```python
from build123d import *

# Parameters (mm, degrees)
SKETCH_1_W          = 300
SKETCH_1_H          = 200
EXTRUDE_1_DEPTH     = 5
SKETCH_3_R          = 1.5
SKETCH_3_R_2        = 2.5
CUT_EXTRUDE_1_DEPTH = 181.346887969


with BuildPart() as part:
    # 草圖1 → 填料-伸長1 (new body)
    with BuildSketch(Plane(origin=(0, 0, 0), x_dir=(1, 0, 0), z_dir=(0, 1, 0))):
        Rectangle(SKETCH_1_W, SKETCH_1_H)
        with BuildLine():
            Line((-137.5, 92.5), (-137.5, 87.5))
            ThreePointArc((-137.5, 87.5), (-140, 85), (-142.5, 87.5))
            Line((-142.5, 87.5), (-142.5, 92.5))
            ThreePointArc((-142.5, 92.5), (-140, 95), (-137.5, 92.5))
        make_face(mode=Mode.SUBTRACT)
        with BuildLine():
            Line((-137.5, 66.785714286), (-137.5, 61.785714286))
            ThreePointArc((-137.5, 61.785714286), (-140, 59.285714286), (-142.5, 61.785714286))
            Line((-142.5, 61.785714286), (-142.5, 66.785714286))
            ThreePointArc((-142.5, 66.785714286), (-140, 69.285714286), (-137.5, 66.785714286))
        make_face(mode=Mode.SUBTRACT)
        with BuildLine():
            Line((-137.5, 41.071428571), (-137.5, 36.071428571))
            ThreePointArc((-137.5, 36.071428571), (-140, 33.571428571), (-142.5, 36.071428571))
            Line((-142.5, 36.071428571), (-142.5, 41.071428571))
            ThreePointArc((-142.5, 41.071428571), (-140, 43.571428571), (-137.5, 41.071428571))
        make_face(mode=Mode.SUBTRACT)
        with BuildLine():
            Line((-137.5, 15.357142857), (-137.5, 10.357142857))
            ThreePointArc((-137.5, 10.357142857), (-140, 7.857142857), (-142.5, 10.357142857))
            Line((-142.5, 10.357142857), (-142.5, 15.357142857))
            ThreePointArc((-142.5, 15.357142857), (-140, 17.857142857), (-137.5, 15.357142857))
        make_face(mode=Mode.SUBTRACT)
        with BuildLine():
            Line((-137.5, -10.357142857), (-137.5, -15.357142857))
            ThreePointArc((-137.5, -15.357142857), (-140, -17.857142857), (-142.5, -15.357142857))
            Line((-142.5, -15.357142857), (-142.5, -10.357142857))
            ThreePointArc((-142.5, -10.357142857), (-140, -7.857142857), (-137.5, -10.357142857))
        make_face(mode=Mode.SUBTRACT)
        with BuildLine():
            Line((-137.5, -36.071428571), (-137.5, -41.071428571))
            ThreePointArc((-137.5, -41.071428571), (-140, -43.571428571), (-142.5, -41.071428571))
            Line((-142.5, -41.071428571), (-142.5, -36.071428571))
            ThreePointArc((-142.5, -36.071428571), (-140, -33.571428571), (-137.5, -36.071428571))
        make_face(mode=Mode.SUBTRACT)
        with BuildLine():
            Line((-137.5, -61.785714286), (-137.5, -66.785714286))
            ThreePointArc((-137.5, -66.785714286), (-140, -69.285714286), (-142.5, -66.785714286))
            Line((-142.5, -66.785714286), (-142.5, -61.785714286))
            ThreePointArc((-142.5, -61.785714286), (-140, -59.285714286), (-137.5, -61.785714286))
        make_face(mode=Mode.SUBTRACT)
        with BuildLine():
            Line((-137.5, -87.5), (-137.5, -92.5))
            ThreePointArc((-137.5, -92.5), (-140, -95), (-142.5, -92.5))
            Line((-142.5, -92.5), (-142.5, -87.5))
            ThreePointArc((-142.5, -87.5), (-140, -85), (-137.5, -87.5))
        make_face(mode=Mode.SUBTRACT)
        with BuildLine():
            Line((137.5, 92.5), (137.5, 87.5))
            ThreePointArc((137.5, 87.5), (140, 85), (142.5, 87.5))
            Line((142.5, 87.5), (142.5, 92.5))
            ThreePointArc((142.5, 92.5), (140, 95), (137.5, 92.5))
        make_face(mode=Mode.SUBTRACT)
        with BuildLine():
            Line((137.5, 66.785714286), (137.5, 61.785714286))
            ThreePointArc((137.5, 61.785714286), (140, 59.285714286), (142.5, 61.785714286))
            Line((142.5, 61.785714286), (142.5, 66.785714286))
            ThreePointArc((142.5, 66.785714286), (140, 69.285714286), (137.5, 66.785714286))
        make_face(mode=Mode.SUBTRACT)
        with BuildLine():
            Line((137.5, 41.071428571), (137.5, 36.071428571))
            ThreePointArc((137.5, 36.071428571), (140, 33.571428571), (142.5, 36.071428571))
            Line((142.5, 36.071428571), (142.5, 41.071428571))
            ThreePointArc((142.5, 41.071428571), (140, 43.571428571), (137.5, 41.071428571))
        make_face(mode=Mode.SUBTRACT)
        with BuildLine():
            Line((-130, -87.5), (130, -87.5))
            ThreePointArc((130, -87.5), (132.5, -90), (130, -92.5))
            Line((130, -92.5), (-130, -92.5))
            ThreePointArc((-130, -92.5), (-132.5, -90), (-130, -87.5))
        make_face(mode=Mode.SUBTRACT)
        with BuildLine():
            Line((-130, 92.5), (130, 92.5))
            ThreePointArc((130, 92.5), (132.5, 90), (130, 87.5))
            Line((130, 87.5), (-130, 87.5))
            ThreePointArc((-130, 87.5), (-132.5, 90), (-130, 92.5))
        make_face(mode=Mode.SUBTRACT)
        with BuildLine():
            Line((137.5, 15.357142857), (137.5, 10.357142857))
            ThreePointArc((137.5, 10.357142857), (140, 7.857142857), (142.5, 10.357142857))
            Line((142.5, 10.357142857), (142.5, 15.357142857))
            ThreePointArc((142.5, 15.357142857), (140, 17.857142857), (137.5, 15.357142857))
        make_face(mode=Mode.SUBTRACT)
        with BuildLine():
            Line((137.5, -10.357142857), (137.5, -15.357142857))
            ThreePointArc((137.5, -15.357142857), (140, -17.857142857), (142.5, -15.357142857))
            Line((142.5, -15.357142857), (142.5, -10.357142857))
            ThreePointArc((142.5, -10.357142857), (140, -7.857142857), (137.5, -10.357142857))
        make_face(mode=Mode.SUBTRACT)
        with BuildLine():
            Line((137.5, -36.071428571), (137.5, -41.071428571))
            ThreePointArc((137.5, -41.071428571), (140, -43.571428571), (142.5, -41.071428571))
            Line((142.5, -41.071428571), (142.5, -36.071428571))
            ThreePointArc((142.5, -36.071428571), (140, -33.571428571), (137.5, -36.071428571))
        make_face(mode=Mode.SUBTRACT)
        with BuildLine():
            Line((137.5, -61.785714286), (137.5, -66.785714286))
            ThreePointArc((137.5, -66.785714286), (140, -69.285714286), (142.5, -66.785714286))
            Line((142.5, -66.785714286), (142.5, -61.785714286))
            ThreePointArc((142.5, -61.785714286), (140, -59.285714286), (137.5, -61.785714286))
        make_face(mode=Mode.SUBTRACT)
        with BuildLine():
            Line((137.5, -87.5), (137.5, -92.5))
            ThreePointArc((137.5, -92.5), (140, -95), (142.5, -92.5))
            Line((142.5, -92.5), (142.5, -87.5))
            ThreePointArc((142.5, -87.5), (140, -85), (137.5, -87.5))
        make_face(mode=Mode.SUBTRACT)
    extrude(amount=EXTRUDE_1_DEPTH)

    # 草圖3 → 除料-伸長1 (cut, through all)
    with BuildSketch(Plane(origin=(0, 5, 0), x_dir=(1, 0, 0), z_dir=(0, 1, 0))):
        with Locations(Location((0, -80.078865529, 0), (0, 0, 270))):
            Circle(SKETCH_3_R)
        with Locations(Location((0, -35.078865529, 0), (0, 0, 270))):
            Circle(SKETCH_3_R)
        with Locations(Location((-98, 14.785714286, 0), (0, 0, 270))):
            Circle(SKETCH_3_R)
        with Locations(Location((-98, 66.785714286, 0), (0, 0, 270))):
            Circle(SKETCH_3_R)
        with Locations(Location((98, 14.785714286, 0), (0, 0, 90))):
            Circle(SKETCH_3_R)
        with Locations(Location((98, 66.785714286, 0), (0, 0, 90))):
            Circle(SKETCH_3_R)
        with Locations(Location((-37.5, 14.421134471, 0), (0, 0, 270))):
            Circle(SKETCH_3_R_2)
    extrude(amount=-CUT_EXTRUDE_1_DEPTH, mode=Mode.SUBTRACT)


solid = part.part
```
Input: part model. Units: mm. Frame: model coordinates. Round coordinates to 2 decimals unless told otherwise and drop trailing zeros. Write each loop counter-clockwise with the first axis right and the second up, starting at its lowest first coordinate (ties: lowest second). Pieces come first, ordered by that corner, then holes. Notation, with made-up numbers: (6.5, 26.5) -> (50.5, 26.5) arc R17 cw to (50.5, 31.5) -> close; hole circle Ø11 at (2, 86). An arc over 180 degrees is marked (long way). Answer as CSV lines item,"result".
1. Ray query, L1, parallel to Z at x = 2, y = 0.85; L2, parallel to Z at x = -98, y = 2.9; L3, parallel to X at y = 0.75, z = -62. Return the intervals inside material, ascending. Write a range as [from, to].
Geometry says:
L1,"z = [-100, -92.5], [-87.5, 87.5], [92.5, 100]"
L2,"z = [-100, -92.5], [-87.5, -68.29], [-65.29, -16.29], [-13.29, 87.5], [92.5, 100]"
L3,"x = [-150, -142.5], [-137.5, 137.5], [142.5, 150]"
2. Contact query for a flat-ended pin moving along its axis: P1, Ø4, axis at x = -98, z = -66.79, coming from the +Y side. Output: stop coordinate, or through.
Geometry says:
P1,"stops at y = 5"
3. Section B-B (y = 2.7). Give the number of separate pieces and of enclosed holes in the cut face, plus the area to 3 significant figures.
Geometry says:
separate pieces,"1"
enclosed holes,"25"
area,"56,600 mm^2"
4. Section A-A (x = 18.5). Return the cut outline in (y, z), plus the area to 3 significant figures.
Geometry says:
outline,"(0, -100) -> (5, -100) -> (5, -92.5) -> (0, -92.5) -> close; (0, -87.5) -> (5, -87.5) -> (5, 87.5) -> (0, 87.5) -> close; (0, 92.5) -> (5, 92.5) -> (5, 100) -> (0, 100) -> close"
area,"950 mm^2"
